from build123d import *

# Parameters (mm, degrees)
F0_W      = 40.5
F0_H      = 28
F1_DEPTH  = 9.8
F2_R      = 6.3
F2_R_2    = 5.1
F3_DEPTH  = 13.4
F3_FACE_R = 5.1
F4_DEPTH  = 9.7
F5_R      = 5
F6_DEPTH  = 2
F7_SIZE   = 0.2


with BuildPart() as f1:
    # F0 (on Front) → F1 (new body)
    with BuildSketch(Plane.XZ):
        with Locations((20.25, -14)):
            Rectangle(F0_W, F0_H)
    extrude(amount=F1_DEPTH)

    # F2 (on face) → F3 (join)
    with BuildSketch(Plane.XZ.offset(9.8)):
        with Locations((23, -14)):
            Circle(F2_R)
        with Locations((23, -14)):
            Circle(F2_R_2, mode=Mode.SUBTRACT)
    extrude(amount=F3_DEPTH)

    # F3_face (on face) → F4 (join)
    with BuildSketch(Plane(origin=(23, -9.8, -14), x_dir=(1, 0, 0), z_dir=(0, -1, 0))):
        Circle(F3_FACE_R)
    extrude(amount=F4_DEPTH)

    # F5 (on face) → F6 (cut)
    with BuildSketch(Plane.XZ.offset(9.8)):
        with Locations((7, -14)):
            Circle(F5_R)
    extrude(amount=-F6_DEPTH, mode=Mode.SUBTRACT)

    # F7
    f7_edges = [f1.edges().sort_by_distance(p)[0] for p in [
        (17.9, -23.2, -14),
        (16.7, -23.2, -14),
    ]]
    chamfer(f7_edges, length=F7_SIZE)


solid = f1.part
Part model, mm, in its own coordinate system. A direction names the side the tool comes from. Coordinates: 2 decimals unless noted, no trailing zeros. Write each loop counter-clockwise with the first axis right and the second up, starting at its lowest first coordinate (ties: lowest second). Pieces come first, ordered by that corner, then holes. Notation, with made-up numbers: M 54.25,-22 L 96.25,-22 A16 cw 96.25,7 Z; hole C 53.25,23 d10. An arc over 180 degrees is marked long. Return JSON: item names as keys, results as strings.
1. Saw through at B-B, the plane x = 7. Write the cut outline in (y, z).
Determined:
{"outline": "M -9.8,-28 L 0,-28 L 0,0 L -9.8,0 L -9.8,-9 L -7.8,-9 L -7.8,-19 L -9.8,-19 Z"}
2. Saw through at A-A, the plane z = -14. Write the cut outline in (x, y), then the cut area to 3 significant figures.
Determined:
{"outline": "M 0,-9.8 L 2,-9.8 L 2,-7.8 L 12,-7.8 L 12,-9.8 L 16.7,-9.8 L 16.7,-23 L 16.9,-23.2 L 17.7,-23.2 L 17.9,-23 L 17.9,-19.5 L 28.1,-19.5 L 28.1,-23 L 28.3,-23.2 L 29.1,-23.2 L 29.3,-23 L 29.3,-9.8 L 40.5,-9.8 L 40.5,0 L 0,0 Z", "area": "508 mm²"}
3. Saw through at D-D, the plane x = 23. Write the cut outline in (y, z), then the cut area to 3 significant figures.
Determined:
{"outline": "M -23.2,-20.1 L -23,-20.3 L -9.8,-20.3 L -9.8,-28 L 0,-28 L 0,0 L -9.8,0 L -9.8,-7.7 L -23,-7.7 L -23.2,-7.9 L -23.2,-8.7 L -23,-8.9 L -19.5,-8.9 L -19.5,-19.1 L -23,-19.1 L -23.2,-19.3 Z", "area": "405 mm²"}
4. 3-axis set-ups, long thin cutter, end or side, ignore diameter. For faces 4 (the face through (18, -23.2, -11)), 5 (the face through (7, -7.8, -14)): which of +Z, -Z, +X, -X, +Y, -Y reach the whole face in a straight line?
Determined:
{"face 4": "+Z, -Z, +X, -X, -Y", "face 5": "-Y"}
5. Pull direction X, two halves, no side cores. Call faces 1 (the face through (20, -5, -28)), 2 (the face through (0, -5, -14)), 3 (the face through (9.307, -8.814, -18.436)): pulls with the +X half, pulls with the -X half, needs draft (parallel to the pull), parting line crosses it, or undercut.
Determined:
{"face 1": "needs draft", "face 2": "pulls with the -X half", "face 3": "undercut"}
6. Saw through at C-C, the plane y = -15. Write the cut outline in (x, z).
Determined:
{"outline": "C 23,-14 d12.6"}
7. Flat gauge pins, fed straight in: pin 1 Ø6 at (x, z) = (7, -14) entering from -Y; pin 2 Ø3 at (x, z) = (21, -25) entering from -Y; pin 3 Ø1 at (x, y) = (30.5, -15.5) entering from -Z; pin 4 Ø3 at (x, z) = (22, -15.5) entering from -Y. Where does each tip first touch, or does it go through?
Determined:
{"pin 1": "y = -7.8", "pin 2": "y = -9.8", "pin 3": "through", "pin 4": "y = -19.5"}
8. Probe L1, parallel to Z at x = 23, y = -20.85; L2, parallel to Y at x = 25.5, z = -12; L3, parallel to Z at x = 27, y = -20.75. List the from-to ranges inside material, lowest first.
Determined:
{"L1": "-20.3 to -19.1, -8.9 to -7.7", "L2": "-19.5 to 0", "L3": "-18.87 to -17.16, -10.84 to -9.13"}
